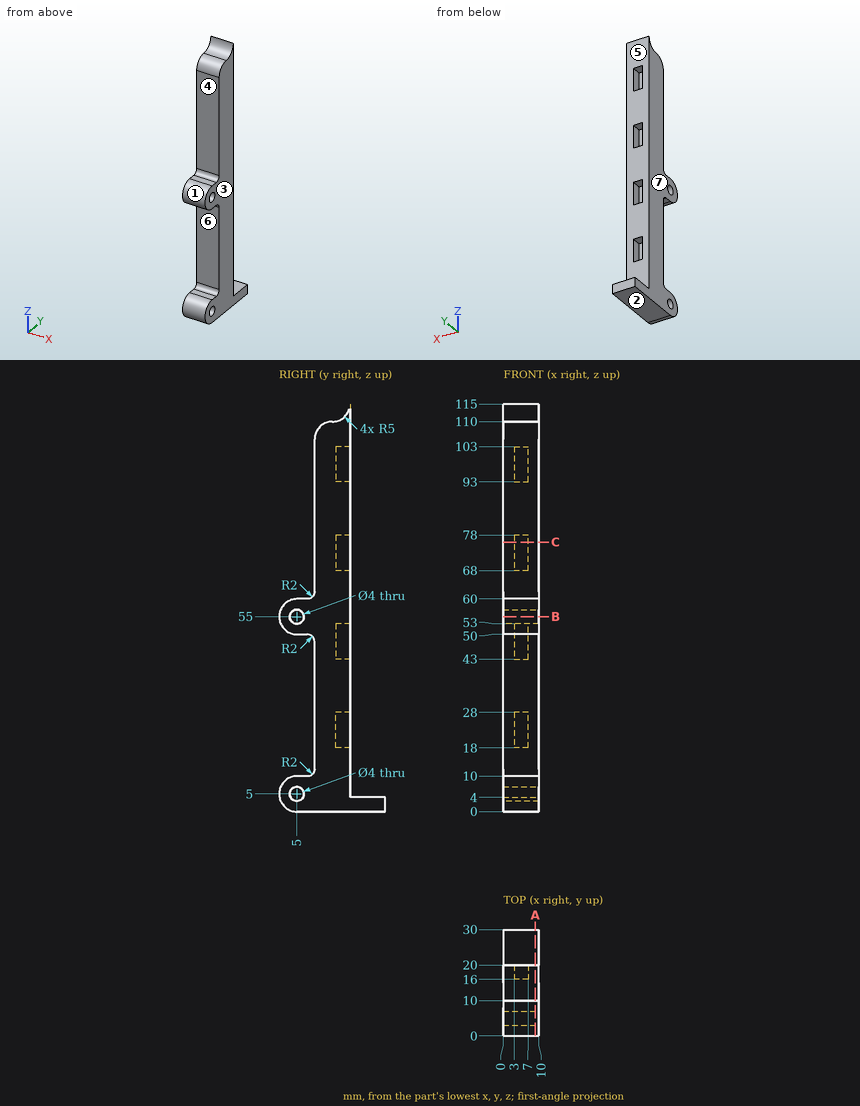
Input: dimensioned drawing with shaded views. Units: mm. Origin: part minimum x, y, z. A direction names the side the tool comes from. Round coordinates to 2 decimals unless told otherwise and drop trailing zeros. Order: outer loops, then holes, each group sorted by start corner. A loop starts at its lowest first (then second) coordinate and runs counter-clockwise, first axis right, second up. Notation, with made-up numbers: M 40,75 L 46,75 A24 ccw 46,90 Z; hole C 38.5,30 d9. An arc over 180 degrees is marked long. Use one line per item in the form item = value. Start each with the question number.
Q1. Cut plane B-B (z = 55). Return loops of the section in (x, y).
Q2. Cut plane A-A (x = 9). Count the separate pieces of the cut face and the enclosed holes in it, and give its area (3 significant figures).
Q3. Material intervals for line 1 (Z direction, x = 7.5, y = 5); line 2 (Y direction, x = 5.5, z = 55); line 3 (X direction, y = 19.25, z = 26.5), sorted ascending. Write a range as [from, to].
Q4. Mould query, pull axis Z, two halves, no side actions, for the marked faces 1, 2 and 3. Classes: +Z half, -Z half, draft (parallel to the pull), parting line (faces both ways), or undercut.
Q5. Access query for the marked faces 4, 5, 6 and 7. Directions: +Z, -Z, +X, -X, +Y, -Y. A direction counts if a zero-diameter tool reaches every point of the face in a straight line with its end or side. Return the directions, or none.
Q6. Pin query (flat end, axial travel): pin 1 Ø4 at (x, z) = (4.5, 82.5) entering from +Y; pin 2 Ø3.5 at (x, y) = (7.5, 6.5) entering from +Z (1 decimal); pin 3 Ø4.5 at (y, z) = (5, 55) entering from -X; pin 4 Ø3 at (x, y) = (4.5, 17) entering from +Z. Return the tip coordinate at first contact, or that it passes through.
Q7. Cut plane C-C (z = 76). Return loops of the section in (x, y).
Geometry results:
q1.outline = M 0,0 L 10,0 L 10,3 L 0,3 Z; M 0,7 L 10,7 L 10,20 L 0,20 Z
q2.separate_pieces = 1
q2.enclosed_holes = 2
q2.area = 1,300 mm^2
q3.line_1 = [0, 3], [7, 10], [50, 53], [57, 60]
q3.line_2 = [0, 3], [7, 20]
q3.line_3 = [0, 3], [7, 10]
q4.face_1 = undercut
q4.face_2 = -Z half
q4.face_3 = draft
q5.face_4 = +Z, +X, -X, -Y
q5.face_5 = +Z, +X, -X, +Y
q5.face_6 = +X, -X, -Y
q5.face_7 = +Z, -Z, -X, +Y, -Y
q6.pin_1 = 20
q6.pin_2 = 60
q6.pin_3 = 0
q6.pin_4 = 111.43
q7.outline = M 0,10 L 10,10 L 10,20 L 7,20 L 7,16 L 3,16 L 3,20 L 0,20 Z
